Here's how the part is built. I have some questions about the finished solid (model axes, mm). A direction names the side the tool comes from. Give positions to 0.01 mm unless a question says otherwise; leave off trailing zeros. Order: outer loops, then holes, each group sorted by start corner. A loop starts at its lowest first (then second) coordinate and runs counter-clockwise, first axis right, second up. Notation, with made-up numbers: (67.5, -18) -> (82.5, -18) arc R20 ccw to (82.5, 9) -> close; hole circle Ø8 at (24, 70.25). An arc over 180 degrees is marked (long way). Write each question's results on one line, items separated by ' | '. Start each with the question number.
Q1. For faces 1 (the face through (11.97, 71.49, 39.05)), 2 (the face through (11, -2, 38)), 3 (the face through (13, -7, 40)), 4 (the face through (11, -2, 42)), which set-ups out of +Z, -Z, +X, -X, +Y, -Y let a thin tool reach every point of the face, with its end or its side?
Q2. Imagine slicing it at A-A, the plane y = -7. Please give me the cut outline in (x, z), then the cut area to 3 significant figures.
Q3. Thinking about a two-plate mould opening in X: for faces 5 (the face through (17, -2, 40)), 6 (the face through (12, -7, 40)), 7 (the face through (12.48, 28.812, 42.343)), 8 (the face through (10.6, -8, 40)), which applies, pulls with the +X half, pulls with the -X half, needs draft (parallel to the pull), parting line crosses it, or undercut?
Q4. I'm going to push flat-ended pins straight in: pin 1 (1.1 mm diameter, centred on x = 12.5, z = 41, fed in from +Y); pin 2 (2 mm diameter, centred on x = 16, y = 44.5, fed in from +Z); pin 3 (1 mm diameter, centred on x = 12, z = 41, fed in from +Y). Where does each tip first touch, or does it pass through?
Q5. I need wall thicknesses on line 1 along X through (y, z) = (-4.5, 41.15); line 2 along X through (y, z) = (8, 40.2); line 3 along Y through (x, z) = (12.5, 39.6). Which ranges of each line are inside material? Lowest first, please. Write a range as [from, to].
Q6. Imagine slicing it at C-C, the plane x = 16.5. Please give me the cut outline in (y, z).
Q7. Imagine slicing it at D-D, the plane y = 54.5. Please give me the cut outline in (x, z), then the cut area to 3 significant figures.
Q8. Imagine slicing it at B-B, the plane y = 67.5. Please give me the cut outline in (x, z).
```python
from build123d import *

# Parameters (mm, degrees)
CYLINDER026_R                                        = 1.4
CYLINDER026_DEPTH                                    = 3
FILLET005011017004_R                                 = 1
BOX085009_W                                          = 1
BOX085009_H                                          = 4.8
BOX085009_DEPTH                                      = 10
BOX085008_W                                          = 7.4
BOX085008_H                                          = 4.8
BOX085008_DEPTH                                      = 11.5
FILLET005011017005_R                                 = 1
FILLET005011017006_R                                 = 4
CYLINDER025_R                                        = 2.4
CYLINDER025_DEPTH                                    = 72.5
CHAMFER011002_SIZE2                                  = 1
CHAMFER011002_SIZE                                   = 10
FUSION004008002002002001007002002008_PLACEMENT_ANGLE = 90


with BuildPart() as fillet005011017004:
    # Cylinder026 → Cylinder026 (new body)
    with BuildSketch(Plane.XY.offset(72.5)):
        Circle(CYLINDER026_R)
    extrude(amount=CYLINDER026_DEPTH)

    # Fillet005011017004
    fillet005011017004_edges = [fillet005011017004.edges().sort_by_distance(p)[0] for p in [
        (-1.4, 0, 75.5),
    ]]
    fillet(fillet005011017004_edges, radius=FILLET005011017004_R)


with BuildPart() as cube097:
    # Box085009 → Box085009 (new body)
    with BuildSketch(Plane(origin=(-1, -2.4, -10), x_dir=(1, 0, 0), z_dir=(0, 0, 1))):
        with Locations((0.5, 2.4)):
            Rectangle(BOX085009_W, BOX085009_H)
    extrude(amount=BOX085009_DEPTH)


with BuildPart() as cut001002016002:
    # Box085008 → Box085008 (new body)
    with BuildSketch(Plane(origin=(-2.4, -2.4, -11.5), x_dir=(1, 0, 0), z_dir=(0, 0, 1))):
        with Locations((3.7, 2.4)):
            Rectangle(BOX085008_W, BOX085008_H)
    extrude(amount=BOX085008_DEPTH)

    # Fillet005011017005
    fillet005011017005_edges = [cut001002016002.edges().sort_by_distance(p)[0] for p in [
        (-2.4, -2.4, -5.75),
        (-2.4, 2.4, -5.75),
    ]]
    fillet(fillet005011017005_edges, radius=FILLET005011017005_R)

    # Fillet005011017006
    fillet005011017006_edges = [cut001002016002.edges().sort_by_distance(p)[0] for p in [
        (5, 0, -11.5),
    ]]
    fillet(fillet005011017006_edges, radius=FILLET005011017006_R)

    # Cut001002016002: cut Cube097
    add(cube097.part, mode=Mode.SUBTRACT)


with BuildPart() as stylus:
    # Cylinder025 → Cylinder025 (new body)
    with BuildSketch(Plane.XY):
        Circle(CYLINDER025_R)
    extrude(amount=CYLINDER025_DEPTH)

    # Chamfer011002
    chamfer011002_edges = [stylus.edges().sort_by_distance(p)[0] for p in [
        (-2.4, 0, 72.5),
    ]]
    chamfer011002_side = stylus.faces().sort_by_distance((-2.4, 0, 36.25))[0]
    chamfer(chamfer011002_edges, length=CHAMFER011002_SIZE, length2=CHAMFER011002_SIZE2, reference=chamfer011002_side)

    # Fusion004008002002002001007002002008: union Fillet005011017004, Cut001002016002
    add(fillet005011017004.part)
    add(cut001002016002.part)


with BuildPart() as stylus_1:
    # Fusion004008002002002001007002002008 placement: moved
    add(stylus.part.moved(Location((13, -2, 40))).rotate(Axis((13, -2, 40), (-1, 0, 0)), FUSION004008002002002001007002002008_PLACEMENT_ANGLE))


solid = stylus_1.part
```
Geometry check:
1) face 1: +Y | face 2: -Z, -X, +Y | face 3: +Z, -Z | face 4: +Z, -X, +Y
2) outline: (10.6, 38.6) arc R1 ccw to (11.6, 37.6) -> (12, 37.6) -> (12, 42.4) -> (11.6, 42.4) arc R1 ccw to (10.6, 41.4) -> close; (13, 37.6) -> (18, 37.6) -> (18, 42.4) -> (13, 42.4) -> close | area: 30.3 mm²
3) face 5: needs draft | face 6: undercut | face 7: parting line crosses it | face 8: pulls with the -X half
4) pin 1: y = 73.49 | pin 2: z = 41.33 | pin 3: y = 73.36
5) line 1: [10.6, 12], [13, 18] | line 2: [10.61, 15.39] | line 3: [-13.5, -12], [-2, 73.47]
6) outline: (-12.62, 37.6) -> (-2, 37.6) -> (-2, 42.4) -> (-12.62, 42.4) -> close
7) outline: circle Ø4.8 at (13, 40) | area: 18.1 mm²
8) outline: circle Ø3.4 at (13, 40)
